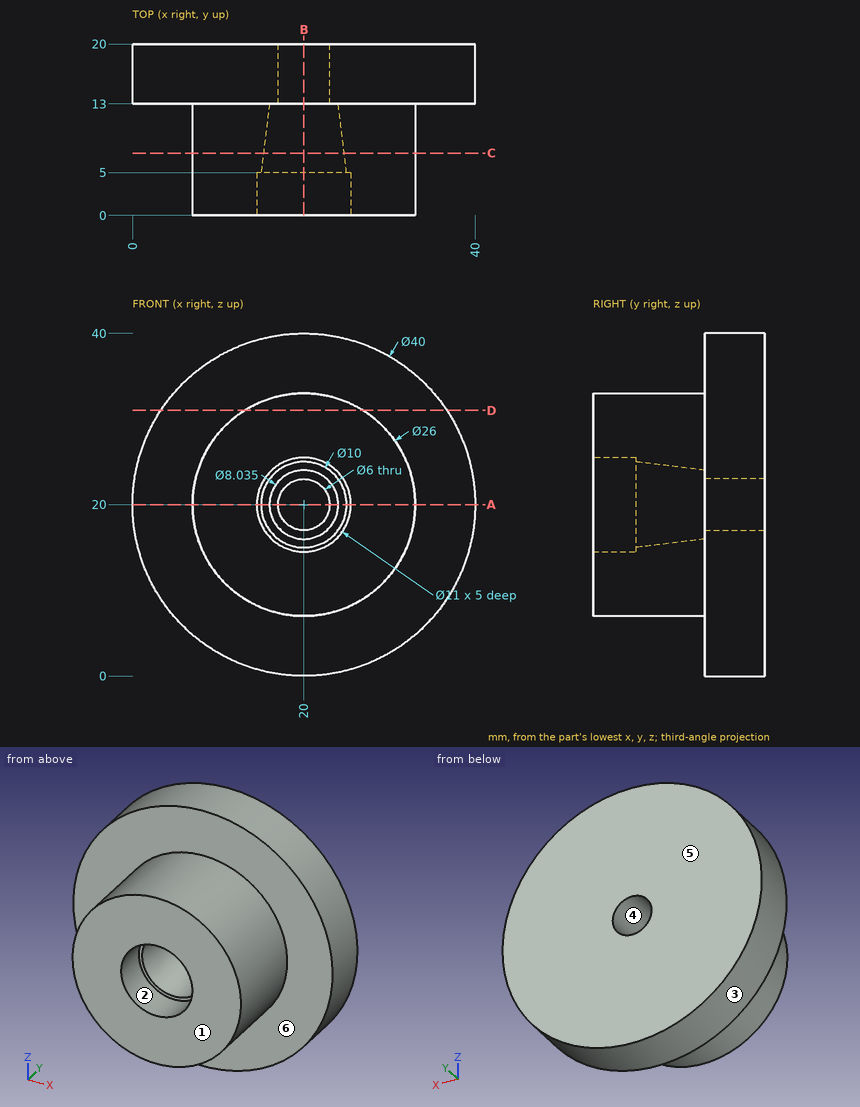
The drawing under review shows one solid part. Ordinate dimensions are in mm from its lowest x, y, z. A direction names the side the tool comes from. Give positions to 0.01 mm unless a question says otherwise; leave off trailing zeros. Write each loop counter-clockwise with the first axis right and the second up, starting at its lowest first coordinate (ties: lowest second). Pieces come first, ordered by that corner, then holes. Notation, with made-up numbers: M 33.5,-5.75 L 42.5,-5.75 A18 cw 42.5,4.25 Z; hole C 27.5,81.25 d8. An arc over 180 degrees is marked long. Write each question's results on one line, items separated by ' | '. Start each with the question number.
1. We need section C-C (y = 7.25). Write out the cut boundary in (x, z), and give its area (3 significant figures).
2. For the marked faces 5 and 6, list the 3-axis set-ups (+Z, -Z, +X, -X, +Y, -Y) from which the entire face can be reached by the end or side of a thin tool; tool diameter is ignored.
3. We need section B-B (x = 20). Write out the cut boundary in (y, z).
4. Mouldability with a two-part tool opening along Z and no side actions: class the marked faces 1, 2, 3 and 4 as released by +Z, released by -Z, zero draft, split by the parting line, or undercut.
5. For probe 1 along X at (y, z) = (15, 20); probe 2 along X at (y, z) = (1.2, 20); probe 3 along Y at (x, z) = (22, 38.5), list the stretches that pass through material, from the lowest coordinate up. Write a range as [from, to].
6. We need section D-D (z = 31). Write out the cut boundary in (x, y), and give its area (3 significant figures).
7. Insertion check: pin 1 Ø5 at (x, z) = (19, 21) entering from +Y; pin 2 Ø8 at (x, y) = (29, 7) entering from +Z; pin 3 Ø6 at (y, z) = (7, 29.5) entering from -X; pin 4 Ø3 at (y, z) = (15.5, 35) entering from -X (1 decimal). Each pin has a flat end and moves straight along its axis. Give the tip position at first contact, or say it passes through.
8. We need section A-A (z = 20). Write out the cut boundary in (x, y).
Results found:
1) outline: C 20,20 d26; hole C 20,20 d9.45 | area: 461 mm^2
2) face 5: +Z, -Z, +X, -X, +Y | face 6: -Y
3) outline: M 0,7 L 13,7 L 13,0 L 20,0 L 20,17 L 13,17 L 13,15.98 L 5,15 L 5,14.5 L 0,14.5 Z; M 0,25.5 L 5,25.5 L 5,25 L 13,24.02 L 13,23 L 20,23 L 20,40 L 13,40 L 13,33 L 0,33 Z
4) face 1: zero draft | face 2: undercut | face 3: split by the parting line | face 4: undercut
5) probe 1: x = [0, 17], [23, 40] | probe 2: x = [7, 14.5], [25.5, 33] | probe 3: y = [13, 20]
6) outline: M 3.3,13 L 13.07,13 L 13.07,0 L 26.93,0 L 26.93,13 L 36.7,13 L 36.7,20 L 3.3,20 Z | area: 414 mm^2
7) pin 1: stops at y = 20 | pin 2: stops at z = 32 | pin 3: stops at x = 8.74 | pin 4: stops at x = 5.2
8) outline: M 0,13 L 7,13 L 7,0 L 14.5,0 L 14.5,5 L 15,5 L 15.98,13 L 17,13 L 17,20 L 0,20 Z; M 23,13 L 24.02,13 L 25,5 L 25.5,5 L 25.5,0 L 33,0 L 33,13 L 40,13 L 40,20 L 23,20 Z
